Here's how the part is built. I have some questions about the finished solid (model axes, mm). A direction names the side the tool comes from. Give positions to 0.01 mm unless a question says otherwise; leave off trailing zeros. Loops run counter-clockwise (first coordinate to the right, second up) from the corner with the lowest first, then second, coordinate; pieces in that order, holes last.
Q1. For faces 1 (the face through (15.1, 2, 23)), 2 (the face through (18, 4, 0)), 3 (the face through (0, 2, -20.1)), which set-ups out of +Z, -Z, +X, -X, +Y, -Y let a thin tool reach every point of the face, with its end or its side?
Q2. I need wall thicknesses on probe 1 along X at (y, z) = (1.15, 20.6); probe 2 along X at (y, z) = (3.15, -20.6); probe 3 along X at (y, z) = (4.85, 15). Which ranges of each line are inside material? Lowest first, please.
Q3. Suppose I cut it at C-C (z = 8.5). List the corners of the cut face in (x, y) for me.
Q4. Suppose I cut it at B-B (x = 28). List the corners of the cut face in (y, z) for me, and give its area (3 significant figures).
Q5. I'm going to push flat-ended pins straight in: P1, Ø4, axis at x = -28, z = -20.6, coming from the +Y side; P2, Ø1, axis at x = 18.5, z = -11.5, coming from the -Y side. Where does each tip first touch, or does it pass through?
Q6. Suppose I cut it at A-A (y = 0.7). Count the separate pieces of the cut face and the enclosed holes in it, and give its area (3 significant figures).
Q7. Suppose I cut it at D-D (x = -2). List the corners of the cut face in (y, z) for me.
Q8. Thinking about a two-plate mould opening in X: for faces 4 (the face through (-33, 2, 0)), 5 (the face through (-18, 4, 0)), 6 (the face through (29.39, 2.46, -19.71)), 7 (the face through (0, 0, 23)), which applies, pulls with the +X half, pulls with the -X half, needs draft (parallel to the pull), parting line crosses it, or undercut?
```python
from build123d import *

# Parameters (mm, degrees)
SKETCH1_W           = 66
SKETCH1_H           = 50
SKETCH1_R           = 1.65
BOSS_EXTRUDE1_DEPTH = 5
SKETCH2_W           = 36
SKETCH2_H           = 36
BOSS_EXTRUDE2_DEPTH = 1.7
CUT_EXTRUDE1_REACH  = 62.117
SKETCH3_W           = 5
SKETCH3_H           = 3.3
FILLET1_R           = 1


with BuildPart() as part:
    # Sketch1 → Boss-Extrude1 (new body)
    with BuildSketch(Plane(origin=(0, 0, 0), x_dir=(1, 0, 0), z_dir=(0, 1, 0))):
        Rectangle(SKETCH1_W, SKETCH1_H)
        with Locations(Location((-28, 20.6, 0), (0, 0, 270))):
            Circle(SKETCH1_R, mode=Mode.SUBTRACT)
        with Locations(Location((28, 20.6, 0), (0, 0, 270))):
            Circle(SKETCH1_R, mode=Mode.SUBTRACT)
        with Locations(Location((-28, -20.6, 0), (0, 0, 270))):
            Circle(SKETCH1_R, mode=Mode.SUBTRACT)
        with Locations(Location((28, -20.6, 0), (0, 0, 270))):
            Circle(SKETCH1_R, mode=Mode.SUBTRACT)
        Polygon((20.1, -20.1), (20.1, 21.1), (18.1, 21.1), (18.1, 20.1), (-18.1, 20.1), (-18.1, 21.1), (-20.1, 21.1), (-20.1, -20.1), align=None, mode=Mode.SUBTRACT)
    extrude(amount=BOSS_EXTRUDE1_DEPTH)

    # Sketch2 → Boss-Extrude2 (add)
    with BuildSketch(Plane(origin=(0, 5, 0), x_dir=(1, 0, 0), z_dir=(0, 1, 0))):
        Polygon((-20.1, 21.1), (-20.1, -20.1), (20.1, -20.1), (20.1, 21.1), (18.1, 21.1), (18.1, 20.1), (-18.1, 20.1), (-18.1, 21.1), align=None)
        Rectangle(SKETCH2_W, SKETCH2_H, mode=Mode.SUBTRACT)
    extrude(amount=-BOSS_EXTRUDE2_DEPTH)

    # Sketch3 → Cut-Extrude1 (cut, up to next)
    with BuildSketch(Plane.XY.offset(25), mode=Mode.PRIVATE) as cut_extrude1_sk1:
        with Locations((-17.6, 1.65)):
            Rectangle(SKETCH3_W, SKETCH3_H)
    cut_extrude1_tool1 = extrude(cut_extrude1_sk1.sketch, amount=-CUT_EXTRUDE1_REACH, mode=Mode.PRIVATE) & part.part
    # Sketch3 → Cut-Extrude1 (cut, up to next)
    with BuildSketch(Plane.XY.offset(25), mode=Mode.PRIVATE) as cut_extrude1_sk2:
        with Locations((17.6, 1.65)):
            Rectangle(SKETCH3_W, SKETCH3_H)
    cut_extrude1_tool2 = extrude(cut_extrude1_sk2.sketch, amount=-CUT_EXTRUDE1_REACH, mode=Mode.PRIVATE) & part.part
    add(cut_extrude1_tool1.solids().sort_by_distance((-17.6, 1.65, 25))[0], mode=Mode.SUBTRACT)
    add(cut_extrude1_tool2.solids().sort_by_distance((17.6, 1.65, 25))[0], mode=Mode.SUBTRACT)

    # Fillet1
    fillet1_edges = [part.edges().sort_by_distance(p)[0] for p in [
        (-18, 4.15, 18),
        (18, 4.15, 18),
        (18, 4.15, -18),
        (-18, 4.15, -18),
        (-20.1, 1.65, -21.1),
        (-18.1, 1.65, -21.1),
        (18.1, 1.65, -21.1),
        (20.1, 1.65, -21.1),
    ]]
    fillet(fillet1_edges, radius=FILLET1_R - 0.0001)  # a hair under: the kernel refuses the full size


solid = part.part
```
Solutions:
1. face 1: +Z, -Y
1. face 2: +Y, -Y
1. face 3: -Y
2. probe 1: x = -33 to -29.65, -26.35 to -20.1, -15.1 to 15.1, 20.1 to 26.35, 29.65 to 33
2. probe 2: x = -33 to -29.65, -26.35 to -19.97, -18.23 to 18.23, 19.97 to 26.35, 29.65 to 33
2. probe 3: x = -33 to -18, 18 to 33
3. outline: (-33, 0) - (-20.1, 0) - (-20.1, 3.3) - (-18, 3.3) - (-18, 5) - (-33, 5) - close; (18, 3.3) - (20.1, 3.3) - (20.1, 0) - (33, 0) - (33, 5) - (18, 5) - close
4. outline: (0, -25) - (5, -25) - (5, -22.25) - (0, -22.25) - close; (0, -18.95) - (5, -18.95) - (5, 18.95) - (0, 18.95) - close; (0, 22.25) - (5, 22.25) - (5, 25) - (0, 25) - close
4. area: 217 mm2
5. P1: stops at y = 5
5. P2: stops at y = 3.3
6. separate pieces: 2
6. enclosed holes: 4
6. area: 1,600 mm2
7. outline: (0, -25) - (5, -25) - (5, -18) - (3.3, -18) - (3.3, -20.1) - (0, -20.1) - close; (0, 20.1) - (3.3, 20.1) - (3.3, 18) - (5, 18) - (5, 25) - (0, 25) - close
8. face 4: pulls with the -X half
8. face 5: undercut
8. face 6: undercut
8. face 7: needs draft
